Geometry check sheet. Reference: the model listing, model coordinates, mm. Face numbers are marked on the shaded views. Give positions to 0.01 mm unless a question says otherwise; leave off trailing zeros. Write each loop counter-clockwise with the first axis right and the second up, starting at its lowest first coordinate (ties: lowest second). Pieces come first, ordered by that corner, then holes. Notation, with made-up numbers: M 5.25,10 L 27.25,10 A22 cw 27.25,40 Z; hole C 59.5,47.5 d11. An arc over 180 degrees is marked long. One line per item, written item: value. Start each with the question number.
1. Cross-section at B-B on x = 10.5. Record the cut outline in (y, z).
2. Cross-section at C-C on y = 5.25. Record the cut outline in (x, z), then the cut area to 3 significant figures.
3. Cross-section at A-A on z = -42. Record the cut outline in (x, y).
4. Release check for a two-part mould opening along Z. For the marked faces 1, 2 and 3 record: pulls with the +Z half, pulls with the -Z half, needs draft (parallel to the pull), parting line crosses it, or undercut.
5. Gauge pin test, flat ends, axial feed: pin 1 (3 mm diameter, centred on y = 0, z = 8.5, fed in from +X); pin 2 (1 mm diameter, centred on y = 8.5, z = -4, fed in from +X); pin 3 (4 mm diameter, centred on x = 6.5, y = 8.5, fed in from +Z). Record the tip position at first contact, or that the pin passes through.
6. Cross-section at D-D on z = 4. Record the cut outline in (x, y).
7. Scan lines: line 1 (Y direction, x = 0, z = -6.5); line 2 (Z direction, x = -9.5, y = 1.5); line 3 (Y direction, x = 8.5, z = -5). Record each from-to range of solid material in increasing order.
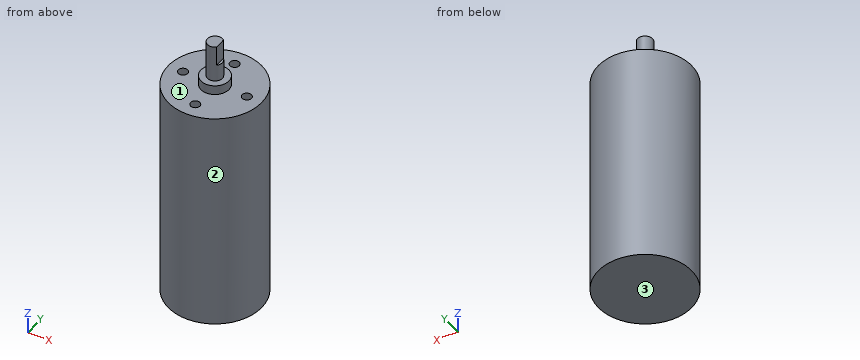
from build123d import *

# Parameters (mm, degrees)
SKETCH1_R                       = 12.5
BOSS_EXTRUDE1_DEPTH             = 60
SKETCH4_R                       = 2
BOSS_EXTRUDE3_DEPTH             = 12.446
SKETCH5_R                       = 3.75
BOSS_EXTRUDE4_DEPTH             = 2.54
CUT_EXTRUDE2_START              = -5.334
CUT_EXTRUDE2_DEPTH              = 5.334
TAP_DRILL_FOR_M3X0_5_TAP1_D     = 2.5
TAP_DRILL_FOR_M3X0_5_TAP1_DEPTH = 10.0000054
TAP_DRILL_FOR_M3X0_5_TAP1_TIP   = 0.751075774


with BuildPart() as part:
    # Sketch1 → Boss-Extrude1 (new body)
    with BuildSketch(Plane.XY):
        Circle(SKETCH1_R)
    extrude(amount=-BOSS_EXTRUDE1_DEPTH)

    # Sketch4 → Boss-Extrude3 (add)
    with BuildSketch(Plane.XY):
        Circle(SKETCH4_R)
    extrude(amount=BOSS_EXTRUDE3_DEPTH)

    # Sketch5 → Boss-Extrude4 (add)
    with BuildSketch(Plane.XY):
        Circle(SKETCH5_R)
    extrude(amount=BOSS_EXTRUDE4_DEPTH)

    # Sketch6 → Cut-Extrude2 (cut)
    with BuildSketch(Plane.XY.offset(12.446).offset(CUT_EXTRUDE2_START)):
        with BuildLine():
            Line((1.35278764, 1.473080311), (1.35278764, -1.473080311))
            ThreePointArc((1.35278764, -1.473080311), (2, 0), (1.35278764, 1.473080311))
        make_face()
    extrude(amount=CUT_EXTRUDE2_DEPTH, mode=Mode.SUBTRACT)

    # Tap Drill for M3x0.5 Tap1
    with Locations(Plane.XY):
        with Locations((0, 8.5), (8.5, 0), (0, -8.5), (-8.5, 0)):
            Hole(TAP_DRILL_FOR_M3X0_5_TAP1_D / 2, depth=TAP_DRILL_FOR_M3X0_5_TAP1_DEPTH)
            with Locations((0, 0, -(TAP_DRILL_FOR_M3X0_5_TAP1_DEPTH + TAP_DRILL_FOR_M3X0_5_TAP1_TIP / 2))):  # 118° drill point
                Cone(0, TAP_DRILL_FOR_M3X0_5_TAP1_D / 2, TAP_DRILL_FOR_M3X0_5_TAP1_TIP, mode=Mode.SUBTRACT)


solid = part.part
Report:
1. outline: M -6.78,-60 L 6.78,-60 L 6.78,0 L -6.78,0 Z
2. outline: M -11.34,-60 L 11.34,-60 L 11.34,0 L -11.34,0 Z
2. area: 1,360 mm^2
3. outline: C 0,0 d25
4. face 1: pulls with the +Z half
4. face 2: needs draft
4. face 3: pulls with the -Z half
5. pin 1: stops at x = 2
5. pin 2: stops at x = 9.6
5. pin 3: stops at z = 0
6. outline: C 0,0 d4
7. line 1: y = -12.5 to -9.75, -7.25 to 7.25, 9.75 to 12.5
7. line 2: z = -60 to 0
7. line 3: y = -9.17 to -1.25, 1.25 to 9.17
